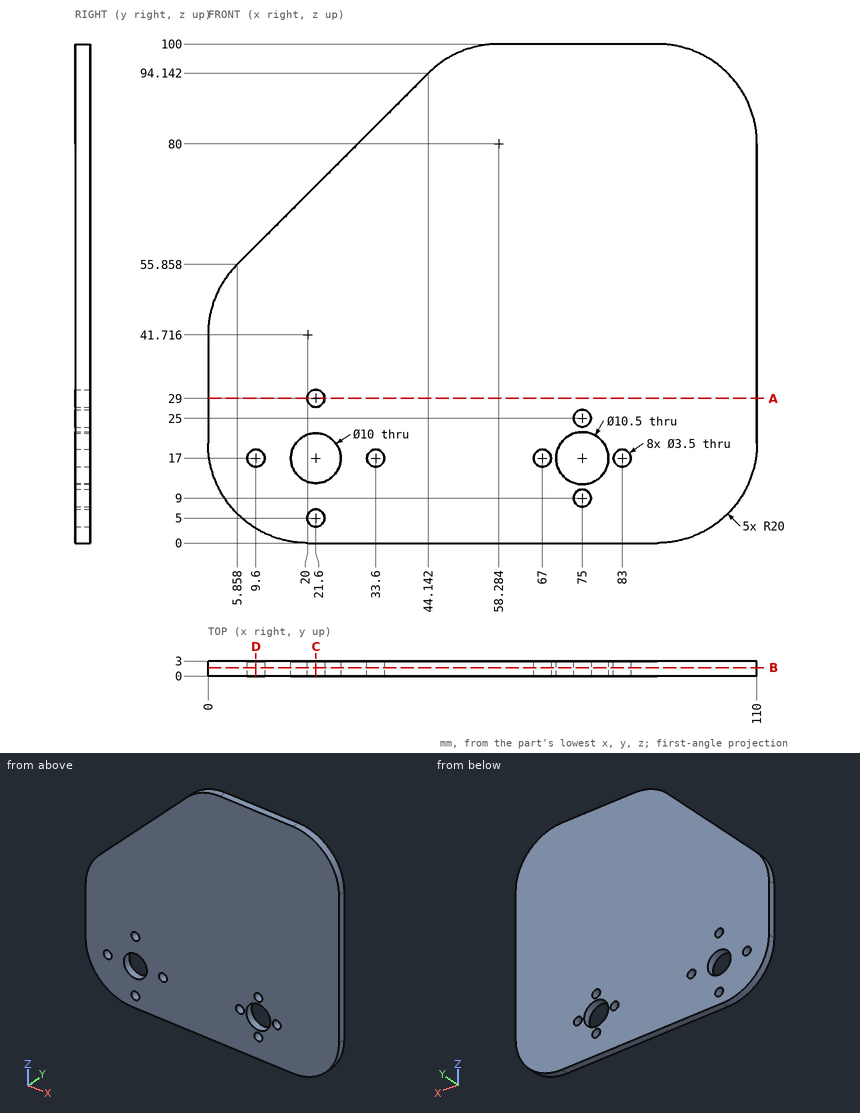
For this review, use the dimensioned drawing (mm, ordinates from the lowest corner) and the shaded views. Give positions to 0.01 mm unless a question says otherwise; leave off trailing zeros. Write each loop counter-clockwise with the first axis right and the second up, starting at its lowest first coordinate (ties: lowest second). Pieces come first, ordered by that corner, then holes. Notation, with made-up numbers: M 50.5,73.5 L 76.5,73.5 A7 cw 76.5,86.5 Z; hole C 75,-25 d9. An arc over 180 degrees is marked long. Answer as a JSON object with one key per item and string values. Group by question number.
Item 1: Consider section B-B on y = 1.7. Count the separate pieces of the cut face and the enclosed holes in it, plus the area to 3 significant figures.
Item 2: For pin 1 Ø3 at (x, z) = (21.6, 29) entering from +Y, flat-tipped, find the tip position at first contact; note if it passes through.
Item 3: Consider section A-A on z = 29. Write out the cut boundary in (x, y).
Item 4: Consider section C-C on x = 21.6. Write out the cut boundary in (y, z).
Item 5: For probe 1 along Z at (x, y) = (75, 0.6); probe 2 along Z at (x, y) = (83, 2); probe 3 along X at (y, z) = (2.25, 25), list the stretches that pass through material, from the lowest coordinate up. Write a range as [from, to].
Item 6: Consider section D-D on x = 9.6. Write out the cut boundary in (y, z).
Check result:
{
 "1": {"separate pieces": "1", "enclosed holes": "10", "area": "9,230 mm^2"},
 "2": {"pin 1": "passes through"},
 "3": {"outline": "M 0,0 L 19.85,0 L 19.85,3 L 0,3 Z; M 23.35,0 L 110,0 L 110,3 L 23.35,3 Z"},
 "4": {"outline": "M 0,0 L 3,0 L 3,3.25 L 0,3.25 Z; M 0,6.75 L 3,6.75 L 3,12 L 0,12 Z; M 0,22 L 3,22 L 3,27.25 L 0,27.25 Z; M 0,30.75 L 3,30.75 L 3,71.6 L 0,71.6 Z"},
 "5": {"probe 1": "z = [0, 7.25], [10.75, 11.75], [22.25, 23.25], [26.75, 100]", "probe 2": "z = [0, 15.25], [18.75, 100]", "probe 3": "x = [0, 73.25], [76.75, 110]"},
 "6": {"outline": "M 0,2.92 L 3,2.92 L 3,15.25 L 0,15.25 Z; M 0,18.75 L 3,18.75 L 3,59.6 L 0,59.6 Z"}
}
